from build123d import *

# Parameters (mm, degrees)
SKETCH_R        = 7.5
SKETCH_R_2      = 4.25
PAD_DEPTH       = 75
SKETCH004_R     = 1.5
HOLE001_DEPTH   = 25
HOLE001_TIPS_R  = 1.5
SKETCH005_R     = 11
POCKET002_DEPTH = 33
SKETCH006_R     = 11
POCKET003_DEPTH = 33


with BuildPart() as part:
    # Sketch → Pad (new body)
    with BuildSketch(Plane.XY):
        with BuildLine():
            ThreePointArc((-38.9, 12.5), (-51.39943, -0.119353), (-38.661306, -12.497721))
            Line((-38.661306, -12.497721), (31.138694, -12.497721))
            ThreePointArc((31.138694, -12.497721), (43.39943, 0.119353), (30.9, 12.5))
            Line((-38.9, 12.5), (30.9, 12.5))
        make_face()
        with Locations((-38.9, 0)):
            Circle(SKETCH_R, mode=Mode.SUBTRACT)
        with Locations((30.9, 0)):
            Circle(SKETCH_R_2, mode=Mode.SUBTRACT)
    extrude(amount=PAD_DEPTH)

    # Sketch004 → Hole001 (cut)
    with BuildSketch(Plane.XZ.offset(12.5)):
        with Locations((1.338694, 72)):
            Circle(SKETCH004_R)
        with Locations((1.338694, 54)):
            Circle(SKETCH004_R)
        with Locations((1.338694, 21)):
            Circle(SKETCH004_R)
        with Locations((1.338694, 3)):
            Circle(SKETCH004_R)
    extrude(amount=-HOLE001_DEPTH, mode=Mode.SUBTRACT)

    # Hole001 tips → Hole001 tip 1 section 0
    with BuildSketch(Plane.XZ.offset(-12.5), mode=Mode.PRIVATE) as hole001_tip_1_s0:
        with Locations((1.338694, 72)):
            Circle(HOLE001_TIPS_R)
    loft([hole001_tip_1_s0.sketch, Vertex(1.338694, 13.401291, 72)], mode=Mode.SUBTRACT)

    # Hole001 tips → Hole001 tip 2 section 0
    with BuildSketch(Plane.XZ.offset(-12.5), mode=Mode.PRIVATE) as hole001_tip_2_s0:
        with Locations((1.338694, 54)):
            Circle(HOLE001_TIPS_R)
    loft([hole001_tip_2_s0.sketch, Vertex(1.338694, 13.401291, 54)], mode=Mode.SUBTRACT)

    # Hole001 tips → Hole001 tip 3 section 0
    with BuildSketch(Plane.XZ.offset(-12.5), mode=Mode.PRIVATE) as hole001_tip_3_s0:
        with Locations((1.338694, 21)):
            Circle(HOLE001_TIPS_R)
    loft([hole001_tip_3_s0.sketch, Vertex(1.338694, 13.401291, 21)], mode=Mode.SUBTRACT)

    # Hole001 tips → Hole001 tip 4 section 0
    with BuildSketch(Plane.XZ.offset(-12.5), mode=Mode.PRIVATE) as hole001_tip_4_s0:
        with Locations((1.338694, 3)):
            Circle(HOLE001_TIPS_R)
    loft([hole001_tip_4_s0.sketch, Vertex(1.338694, 13.401291, 3)], mode=Mode.SUBTRACT)

    # Sketch005 (on Face5 of Hole001) → Pocket002 (cut)
    with BuildSketch(Plane.XY.offset(75)):
        with Locations((30.9, 0)):
            Circle(SKETCH005_R)
    extrude(amount=-POCKET002_DEPTH, mode=Mode.SUBTRACT)

    # Sketch006 (on Face4 of Pocket002) → Pocket003 (cut)
    with BuildSketch(Plane(origin=(0, 0, 0), x_dir=(1, 0, 0), z_dir=(0, 0, -1))):
        with Locations((30.9, 0)):
            Circle(SKETCH006_R)
    extrude(amount=-POCKET003_DEPTH, mode=Mode.SUBTRACT)


solid = part.part
The model under review builds one solid part; all positions refer to its coordinate system, in mm. A direction names the side the tool comes from. Give positions to 0.01 mm unless a question says otherwise; leave off trailing zeros. Write each loop counter-clockwise with the first axis right and the second up, starting at its lowest first coordinate (ties: lowest second). Pieces come first, ordered by that corner, then holes.
1. Add section A-A, the plane z = 72. Write out the cut boundary in (x, y), plus the area to 3 significant figures.
2. Tool access review of faces 1 (the flat face through (31, 5, 33)), 2 (the cylindrical face through (-46.393, 0.33, 36.975)), 3 (the flat face through (31, -5, 42)): name each direction out of +Z, -Z, +X, -X, +Y, -Y from which nothing blocks a thin tool from reaching the whole face with its end or side.
3. For P1, Ø12, axis at x = 25.5, y = 6, coming from the +Z side; P2, Ø6.5, axis at x = 30.5, y = -3, coming from the -Z side; P3, Ø10, axis at y = -8, z = 23.5, coming from the -X side; P4, Ø4, axis at x = 1.34, z = 54, coming from the -Y side, all flat-tipped, find the tip position at first contact; note any pin that passes through.
4. Add section B-B, the plane y = 0. Write out the cut boundary in (x, z).
5. Draft analysis for pull direction Z (two halves, no side actions). For faces 4 (the flat face through (-4, -12.498, 37)), 5 (the flat face through (-15, 0, 75)), 6 (the cylindrical face through (2.15, -0.17, 73.26)), state which applies: +Z half, -Z half, draft (parallel to the pull), parting line (faces both ways), or undercut.
6. Wall thickness on L1, parallel to X at y = -2, z = 17.5; L2, parallel to X at y = 3.5, z = 15; L3, parallel to Y at x = -14.5, z = 5.5: over which ranges is each line inside the solid? List them lowest first.
7. Add section D-D, the plane z = 17. Write out the cut boundary in (x, y).
8. Add section C-C, the plane z = 40. Write out the cut boundary in (x, y).
Worked answers:
1. outline: (-38.9, 12.5) arc R12.5 ccw (long way) to (-38.66, -12.5) - (-0.16, -12.5) - (-0.16, 12.5) - close; (2.84, -12.5) - (31.14, -12.5) arc R12.5 ccw to (30.9, 12.5) - (2.84, 12.5) - close; hole circle Ø15 at (-38.9, 0); hole circle Ø22 at (30.9, 0)
1. area: 1,600 mm2
2. face 1: -Z
2. face 2: +Z, -Z
2. face 3: +Z
3. P1: stops at z = 75
3. P2: stops at z = 33
3. P3: stops at x = -51.03
3. P4: stops at y = -12.5
4. outline: (-51.4, 0) - (-46.4, 0) - (-46.4, 75) - (-51.4, 75) - close; (-31.4, 0) - (19.9, 0) - (19.9, 33) - (26.65, 33) - (26.65, 42) - (19.9, 42) - (19.9, 75) - (-31.4, 75) - close; (35.15, 33) - (41.9, 33) - (41.9, 0) - (43.4, 0) - (43.4, 75) - (41.9, 75) - (41.9, 42) - (35.15, 42) - close; hole circle Ø3 at (1.34, 3); hole circle Ø3 at (1.34, 21); hole circle Ø3 at (1.34, 54); hole circle Ø3 at (1.34, 72)
5. face 4: draft
5. face 5: +Z half
5. face 6: undercut
6. L1: x = -51.24 to -46.13, -31.67 to 20.08, 41.72 to 43.24
6. L2: x = -50.9 to -45.53, -32.27 to 20.47, 41.33 to 42.9
6. L3: y = -12.5 to 12.5
7. outline: (-38.9, 12.5) arc R12.5 ccw (long way) to (-38.66, -12.5) - (31.14, -12.5) arc R12.5 ccw to (30.9, 12.5) - close; hole circle Ø15 at (-38.9, 0); hole circle Ø22 at (30.9, 0)
8. outline: (-38.9, 12.5) arc R12.5 ccw (long way) to (-38.66, -12.5) - (31.14, -12.5) arc R12.5 ccw to (30.9, 12.5) - close; hole circle Ø15 at (-38.9, 0); hole circle Ø8.5 at (30.9, 0)
